Source: CAD feature listing. Evaluate the final solid. Frame: model axes, mm. A direction names the side the tool comes from. Give positions to 0.01 mm unless a question says otherwise; leave off trailing zeros. Loops run counter-clockwise (first coordinate to the right, second up) from the corner with the lowest first, then second, coordinate; pieces in that order, holes last. Notation, with made-up numbers: (67.5, 63.25) -> (76.5, 63.25) arc R16 ccw to (76.5, 67.25) -> close; hole circle Ø1 at (-12, -20.5). An arc over 180 degrees is marked (long way). Return JSON: item names as keys, results as strings. Group by question number.
(1) Cut plane A-A on z = -46.5. Return loops of the section in (x, y) (3 decimals), then the cut area to 3 significant figures.
(2) Ray query, line 1 (X direction, y = 2.5, z = -5); line 2 (Z direction, x = 31.5, y = -1); line 3 (Y direction, x = 0, z = -72) (3 decimals). Return the intervals inside material, ascending. Write a range as from..to.
(3) Cut plane B-B on z = 36.5. Return loops of the section in (x, y) (3 decimals).
(4) Pin query (flat end, axial travel): pin 1 (3 mm diameter, centred on x = 25, y = 0.5, fed in from +Z); pin 2 (3.5 mm diameter, centred on x = -13.42, z = -7.75, fed in from -Y); pin 3 (1 mm diameter, centred on x = -13, y = 0, fed in from -Z); pin 4 (3 mm diameter, centred on x = 34, y = 0.5, fed in from -Z). Return the tip coordinate at first contact, or that it passes through.
(5) Access query for faces 4 (the face through (13.85, 0, -40)), 5 (the face through (-7.5, 0, -23)), 6 (the face through (-8.45, -0.04, -45.91)). Directions: +Z, -Z, +X, -X, +Y, -Y. A direction counts if a zero-diameter tool reaches every point of the face in a straight line with its end or side. Return the directions, or none.
(6) Draft query along Z for faces 1 (the face through (25, 3.175, -9)), 2 (the face through (-13, 0, -15)), 3 (the face through (28.837, 0.044, 39.444)). Return one class per face: released by +Z, released by -Z, zero draft, split by the parting line, or undercut.
```python
from build123d import *

# Parameters (mm, degrees)
SKETCH1_R                                       = 7.5
BOSS_EXTRUDE1_DEPTH                             = 3.175
M5X0_8_TAPPED_HOLE2_D                           = 4.2
CIRPATTERN1_COUNT                               = 3
CIRPATTERN1_ANGLE                               = 135
M3_CLEARANCE_HOLE1_D                            = 3.2
M3_CLEARANCE_HOLE1_DEPTH                        = 15
CSK_FOR_M3_FLAT_HEAD_MACHINE_SCREW1_D           = 3.2
CSK_FOR_M3_FLAT_HEAD_MACHINE_SCREW1_CSINK_D     = 6.3
CSK_FOR_M3_FLAT_HEAD_MACHINE_SCREW1_CSINK_ANGLE = 90
M3X0_5_TAPPED_HOLE1_D                           = 2.5
CUT_EXTRUDE1_REACH                              = 107.268
FILLET1_R                                       = 3.175
F_1_4_CLEARANCE_HOLE1_D                         = 6.7564


with BuildPart() as part:
    # Sketch1 → Boss-Extrude1 (new, symmetric)
    with BuildSketch(Plane(origin=(0, 0, 0), x_dir=(1, 0, 0), z_dir=(0, 1, 0))):
        with BuildLine():
            Line((-13.85, 35), (-7.5, 35))
            Line((-7.5, 35), (-7.5, 15))
            Line((-7.5, 15), (-16.770509831, 15))
            ThreePointArc((-16.770509831, 15), (-18.002512666, -13.496649128), (9.696699141, -20.303300859))
            Line((9.696699141, -20.303300859), (46.966384428, -57.572986146))
            ThreePointArc((46.966384428, -57.572986146), (68.644249266, 28.433379025), (-7.5, 73.920497834))
            Line((-7.5, 73.920497834), (-7.5, 45))
            Line((-7.5, 45), (-13.85, 45))
            Line((-13.85, 45), (-13.85, 35))
        make_face()
        with Locations(Location((0, 0, 0), (0, 0, 270))):
            Circle(SKETCH1_R, mode=Mode.SUBTRACT)
        with BuildLine():
            Line((20.303300859, -9.696699141), (46.898012061, -36.291410343))
            ThreePointArc((46.898012061, -36.291410343), (58.160567128, -11.568856096), (57.216234934, 15.581798996))
            Line((57.216234934, 15.581798996), (22.468570216, 1.188845008))
            ThreePointArc((22.468570216, 1.188845008), (22.067668809, -4.389532245), (20.303300859, -9.696699141))
        make_face(mode=Mode.SUBTRACT)
        with BuildLine():
            Line((7.5, 15), (7.5, 35))
            Line((7.5, 35), (13.85, 35))
            Line((13.85, 35), (13.85, 45))
            Line((13.85, 45), (7.5, 45))
            Line((7.5, 45), (7.5, 58.823804705))
            ThreePointArc((7.5, 58.823804705), (32.945314818, 49.30614801), (51.475983449, 29.439991983))
            Line((51.475983449, 29.439991983), (16.72831873, 15.047037996))
            Line((16.72831873, 15.047037996), (16.614758962, 15))
            Line((16.614758962, 15), (7.5, 15))
        make_face(mode=Mode.SUBTRACT)
    extrude(amount=BOSS_EXTRUDE1_DEPTH, both=True)

    # M5x0.8 Tapped Hole2 (through all)
    with Locations(Plane(origin=(0, 3.175, 0), x_dir=(1, 0, 0), z_dir=(0, 1, 0))):
        with Locations((0, -15.5), (-13.423393759, 7.75), (13.423393759, 7.75)):
            Hole(M5X0_8_TAPPED_HOLE2_D / 2)

    # Sketch5 → M2.5x0.45 Tapped Hole1 (revolve, cut)
    with BuildSketch(Plane(origin=(0, 0, -74.3), x_dir=(0, 1, 0), z_dir=(1, 0, 0))):
        Polygon((0, 0), (0, 10.615882135), (1.025, 10), (1.025, 0), align=None)
    m2_5x0_45_tapped_hole1 = revolve(axis=Axis((0, 0, -80.65), (0, 0, 1)), mode=Mode.SUBTRACT)

    # CirPattern1: M2.5x0.45 Tapped Hole1 ×3 about axis
    cirpattern1_axis = Axis((0, 3.175, 0), (0, -1, 0))
    for i in range(1, CIRPATTERN1_COUNT):
        add(m2_5x0_45_tapped_hole1.rotate(cirpattern1_axis, i * CIRPATTERN1_ANGLE / (CIRPATTERN1_COUNT - 1)), mode=Mode.SUBTRACT)

    # M3 Clearance Hole1
    with Locations(Plane.ZY.offset(7.5)):
        with Locations((-25, 0)):
            Hole(M3_CLEARANCE_HOLE1_D / 2, depth=M3_CLEARANCE_HOLE1_DEPTH)

    # CSK for M3 Flat Head Machine Screw1 (through all)
    with Locations(Plane(origin=(0, -3.175, 0), x_dir=(-1, 0, 0), z_dir=(0, -1, 0))):
        with Locations((-37.112091566, 55.542170102), (-65.516456731, -13.032033511)):
            CounterSinkHole(CSK_FOR_M3_FLAT_HEAD_MACHINE_SCREW1_D / 2, CSK_FOR_M3_FLAT_HEAD_MACHINE_SCREW1_CSINK_D / 2, counter_sink_angle=CSK_FOR_M3_FLAT_HEAD_MACHINE_SCREW1_CSINK_ANGLE)

    # M3x0.5 Tapped Hole1 (through all)
    with Locations(Plane(origin=(0, -3.175, 0), x_dir=(-1, 0, 0), z_dir=(0, -1, 0))):
        with Locations((-31.819805153, -31.819805153)):
            Hole(M3X0_5_TAPPED_HOLE1_D / 2)

    # Sketch12 → Cut-Extrude1 (cut, up to next)
    with BuildSketch(Plane(origin=(0, 3.175, 0), x_dir=(1, 0, 0), z_dir=(0, 1, 0)), mode=Mode.PRIVATE) as cut_extrude1_sk1:
        with BuildLine():
            ThreePointArc((-7.035032015, 16.122532015), (-7.155873257, 16.730041964), (-7.5, 17.24506403))
            Line((-7.5, 17.24506403), (-7.5, 16.122532015))
            Line((-7.5, 16.122532015), (-7.5, 15))
            ThreePointArc((-7.5, 15), (-7.155873257, 15.515022066), (-7.035032015, 16.122532015))
        make_face()
    cut_extrude1_tool1 = extrude(cut_extrude1_sk1.sketch, amount=-CUT_EXTRUDE1_REACH, mode=Mode.PRIVATE) & part.part
    # Sketch12 → Cut-Extrude1 (cut, up to next)
    with BuildSketch(Plane(origin=(0, 3.175, 0), x_dir=(1, 0, 0), z_dir=(0, 1, 0)), mode=Mode.PRIVATE) as cut_extrude1_sk2:
        with BuildLine():
            Line((-8.622532015, 15), (-9.74506403, 15))
            ThreePointArc((-9.74506403, 15), (-8.622532015, 14.535032015), (-7.5, 15))
            Line((-7.5, 15), (-8.622532015, 15))
        make_face()
    cut_extrude1_tool2 = extrude(cut_extrude1_sk2.sketch, amount=-CUT_EXTRUDE1_REACH, mode=Mode.PRIVATE) & part.part
    # Sketch12 → Cut-Extrude1 (cut, up to next)
    with BuildSketch(Plane(origin=(0, 3.175, 0), x_dir=(1, 0, 0), z_dir=(0, 1, 0)), mode=Mode.PRIVATE) as cut_extrude1_sk3:
        with BuildLine():
            Line((8.622532015, 15), (7.5, 15))
            ThreePointArc((7.5, 15), (8.622532015, 14.535032015), (9.74506403, 15))
            Line((9.74506403, 15), (8.622532015, 15))
        make_face()
    cut_extrude1_tool3 = extrude(cut_extrude1_sk3.sketch, amount=-CUT_EXTRUDE1_REACH, mode=Mode.PRIVATE) & part.part
    # Sketch12 → Cut-Extrude1 (cut, up to next)
    with BuildSketch(Plane(origin=(0, 3.175, 0), x_dir=(1, 0, 0), z_dir=(0, 1, 0)), mode=Mode.PRIVATE) as cut_extrude1_sk4:
        with BuildLine():
            Line((7.5, 16.122532015), (7.5, 17.24506403))
            ThreePointArc((7.5, 17.24506403), (7.035032015, 16.122532015), (7.5, 15))
            Line((7.5, 15), (7.5, 16.122532015))
        make_face()
    cut_extrude1_tool4 = extrude(cut_extrude1_sk4.sketch, amount=-CUT_EXTRUDE1_REACH, mode=Mode.PRIVATE) & part.part
    # Sketch12 → Cut-Extrude1 (cut, up to next)
    with BuildSketch(Plane(origin=(0, 3.175, 0), x_dir=(1, 0, 0), z_dir=(0, 1, 0)), mode=Mode.PRIVATE) as cut_extrude1_sk5:
        with BuildLine():
            Line((7.5, 33.877467985), (7.5, 35))
            ThreePointArc((7.5, 35), (7.035032015, 33.877467985), (7.5, 32.75493597))
            Line((7.5, 32.75493597), (7.5, 33.877467985))
        make_face()
    cut_extrude1_tool5 = extrude(cut_extrude1_sk5.sketch, amount=-CUT_EXTRUDE1_REACH, mode=Mode.PRIVATE) & part.part
    # Sketch12 → Cut-Extrude1 (cut, up to next)
    with BuildSketch(Plane(origin=(0, 3.175, 0), x_dir=(1, 0, 0), z_dir=(0, 1, 0)), mode=Mode.PRIVATE) as cut_extrude1_sk6:
        with BuildLine():
            ThreePointArc((9.74506403, 35), (8.622532015, 35.464967985), (7.5, 35))
            Line((7.5, 35), (8.622532015, 35))
            Line((8.622532015, 35), (9.74506403, 35))
        make_face()
    cut_extrude1_tool6 = extrude(cut_extrude1_sk6.sketch, amount=-CUT_EXTRUDE1_REACH, mode=Mode.PRIVATE) & part.part
    # Sketch12 → Cut-Extrude1 (cut, up to next)
    with BuildSketch(Plane(origin=(0, 3.175, 0), x_dir=(1, 0, 0), z_dir=(0, 1, 0)), mode=Mode.PRIVATE) as cut_extrude1_sk7:
        with BuildLine():
            ThreePointArc((-7.035032015, 33.877467985), (-7.155873257, 34.484977934), (-7.5, 35))
            Line((-7.5, 35), (-7.5, 33.877467985))
            Line((-7.5, 33.877467985), (-7.5, 32.75493597))
            ThreePointArc((-7.5, 32.75493597), (-7.155873257, 33.269958036), (-7.035032015, 33.877467985))
        make_face()
    cut_extrude1_tool7 = extrude(cut_extrude1_sk7.sketch, amount=-CUT_EXTRUDE1_REACH, mode=Mode.PRIVATE) & part.part
    # Sketch12 → Cut-Extrude1 (cut, up to next)
    with BuildSketch(Plane(origin=(0, 3.175, 0), x_dir=(1, 0, 0), z_dir=(0, 1, 0)), mode=Mode.PRIVATE) as cut_extrude1_sk8:
        with BuildLine():
            Line((-8.622532015, 35), (-7.5, 35))
            ThreePointArc((-7.5, 35), (-8.622532015, 35.464967985), (-9.74506403, 35))
            Line((-9.74506403, 35), (-8.622532015, 35))
        make_face()
    cut_extrude1_tool8 = extrude(cut_extrude1_sk8.sketch, amount=-CUT_EXTRUDE1_REACH, mode=Mode.PRIVATE) & part.part
    add(cut_extrude1_tool1.solids().sort_by_distance((-7.311461, 3.175, -16.122532))[0], mode=Mode.SUBTRACT)
    add(cut_extrude1_tool2.solids().sort_by_distance((-8.622532, 3.175, -14.811461))[0], mode=Mode.SUBTRACT)
    add(cut_extrude1_tool3.solids().sort_by_distance((8.622532, 3.175, -14.811461))[0], mode=Mode.SUBTRACT)
    add(cut_extrude1_tool4.solids().sort_by_distance((7.311461, 3.175, -16.122532))[0], mode=Mode.SUBTRACT)
    add(cut_extrude1_tool5.solids().sort_by_distance((7.311461, 3.175, -33.877468))[0], mode=Mode.SUBTRACT)
    add(cut_extrude1_tool6.solids().sort_by_distance((8.622532, 3.175, -35.188539))[0], mode=Mode.SUBTRACT)
    add(cut_extrude1_tool7.solids().sort_by_distance((-7.311461, 3.175, -33.877468))[0], mode=Mode.SUBTRACT)
    add(cut_extrude1_tool8.solids().sort_by_distance((-8.622532, 3.175, -35.188539))[0], mode=Mode.SUBTRACT)

    # Fillet1
    fillet1_edges = [part.edges().sort_by_distance(p)[0] for p in [
        (-7.5, 0, -45),
        (9.696699141, 0, 20.303300859),
        (7.5, 0, -58.823804705),
        (7.5, 0, -45),
        (16.614758962, 0, -15),
        (51.475983449, 0, -29.439991983),
        (46.898012061, 0, 36.291410343),
        (57.216234934, 0, -15.581798996),
        (22.468570216, 0, -1.188845008),
        (20.303300859, 0, 9.696699141),
    ]]
    fillet(fillet1_edges, radius=FILLET1_R)

    # 1/4 Clearance Hole1 (through all)
    with Locations(Plane(origin=(0, 3.175, 0), x_dir=(1, 0, 0), z_dir=(0, 1, 0))):
        with Locations((60.541360174, -28.230899884)):
            Hole(F_1_4_CLEARANCE_HOLE1_D / 2)


solid = part.part
```
Answers:
{
 "1": {"outline": "(-7.978, -3.175) -> (7.978, -3.175) -> (7.978, 3.175) -> (-7.978, 3.175) -> close; (36.8, -3.175) -> (57.95, -3.175) -> (57.95, 3.175) -> (36.8, 3.175) -> close", "area": "236 mm²"},
 "2": {"line 1": "-21.94..-5.59, 5.59..31.67, 59.09..74.13", "line 2": "-67.29..-50.24, -21.17..-4.93, 20.89..30.61, 33.03..42.11", "line 3": "-3.175..-1.025, 1.025..3.175"},
 "3": {"outline": "(25.893, -3.175) -> (64.717, -3.175) -> (64.717, 3.175) -> (25.893, 3.175) -> close"},
 "4": {"pin 1": "z = 37.11", "pin 2": "through", "pin 3": "z = -45", "pin 4": "z = -66.81"},
 "5": {"face 4": "+Y, -Y", "face 5": "-X, +Y, -Y", "face 6": "-Z, -X, +Y, -Y"},
 "6": {"face 1": "zero draft", "face 2": "undercut", "face 3": "released by +Z"}
}
